Verification items for the finished model (mm, model axes). A direction names the side the tool comes from. Give positions to 0.01 mm unless a question says otherwise; leave off trailing zeros. Write each loop counter-clockwise with the first axis right and the second up, starting at its lowest first coordinate (ties: lowest second). Pieces come first, ordered by that corner, then holes.
from build123d import *

# Parameters (mm, degrees)
SKETCH1_W           = 38
SKETCH1_H           = 22
BOSS_EXTRUDE1_DEPTH = 18
FILLET1_R           = 5
BOSS_EXTRUDE2_DEPTH = 15
BOSS_EXTRUDE3_DEPTH = 13
FILLET2_R           = 2
SKETCH5_R           = 3
SKETCH5_R_2         = 1.5
CUT_EXTRUDE1_DEPTH  = 52.516987581


with BuildPart() as part:
    # Sketch1 → Boss-Extrude1 (new body)
    with BuildSketch(Plane(origin=(0, 0, 0), x_dir=(0, 0, -1), z_dir=(1, 0, 0))):
        Rectangle(SKETCH1_W, SKETCH1_H)
    extrude(amount=BOSS_EXTRUDE1_DEPTH)

    # Fillet1
    fillet1_edges = [part.edges().sort_by_distance(p)[0] for p in [
        (9, 11, 19),
        (9, -11, 19),
    ]]
    fillet(fillet1_edges, radius=FILLET1_R)

    # Sketch3 → Boss-Extrude2 (add)
    with BuildSketch(Plane(origin=(0, 0, -19), x_dir=(-1, 0, 0), z_dir=(0, 0, -1))):
        with BuildLine():
            Line((-18, 6.32455532), (-18, -6.32455532))
            ThreePointArc((-18, -6.32455532), (-9, -11), (0, -6.32455532))
            Line((0, -6.32455532), (0, 6.32455532))
            ThreePointArc((0, 6.32455532), (-9, 11), (-18, 6.32455532))
        make_face()
    extrude(amount=BOSS_EXTRUDE2_DEPTH)

    # Sketch4 → Boss-Extrude3 (add)
    with BuildSketch(Plane(origin=(0, 0, -34), x_dir=(-1, 0, 0), z_dir=(0, 0, -1))):
        with BuildLine():
            Line((-17, 6), (-17, -6))
            ThreePointArc((-17, -6), (-9, -10), (-1, -6))
            Line((-1, -6), (-1, 6))
            ThreePointArc((-1, 6), (-9, 10), (-17, 6))
        make_face()
    extrude(amount=BOSS_EXTRUDE3_DEPTH)

    # Fillet2
    fillet2_edges = [part.edges().sort_by_distance(p)[0] for p in [
        (9, 10, -47),
        (9, -10, -47),
    ]]
    fillet(fillet2_edges, radius=FILLET2_R - 0.0001)  # a hair under: the kernel refuses the full size

    # Sketch5 → Cut-Extrude1 (cut, through all)
    with BuildSketch(Plane(origin=(18, 0, 0), x_dir=(0, 0, -1), z_dir=(1, 0, 0))):
        with Locations((-8, 0)):
            Circle(SKETCH5_R)
        with Locations((14, -9)):
            Circle(SKETCH5_R_2)
        with Locations(Location((14, 9, 0), (0, 0, 180))):
            Circle(SKETCH5_R_2)
    extrude(amount=-CUT_EXTRUDE1_DEPTH, mode=Mode.SUBTRACT)


solid = part.part
Item 1: Release check for a two-part mould opening along Y. For faces 5 (the face through (9, 11, -26)), 6 (the face through (9.1, -9.9, -12.8)), 7 (the face through (2, -10, -19)) record: released by +Y, released by -Y, zero draft, split by the parting line, or undercut.
Answer key:
face 5: released by +Y
face 6: undercut
face 7: zero draft
Item 2: Sectioned sample at D-D on z = -24. Record the cut outline in (x, y), then the cut area to 3 significant figures.
Answer key:
outline: (0, -6.32) arc R11 ccw to (18, -6.32) - (18, 6.32) arc R11 ccw to (0, 6.32) - close
area: 346 mm2
Item 3: Sectioned sample at A-A on z = 8. Record the cut outline in (x, y).
Answer key:
outline: (0, -11) - (18, -11) - (18, -3) - (0, -3) - close; (0, 3) - (18, 3) - (18, 11) - (0, 11) - close
Item 4: Depth check by flat-ended pin: pin 1 (2.5 mm diameter, centred on x = 13, y = -8.5, fed in from -Z); pin 2 (1.4 mm diameter, centred on x = 6, y = 9, fed in from -Z); pin 3 (5 mm diameter, centred on x = 14, y = -7.5, fed in from +Z); pin 4 (4 mm diameter, centred on x = 4, z = -30.5, fed in from +Y). Enter the tip coordinate at first touch or a pass-through.
Answer key:
pin 1: stops at z = -46.99
pin 2: stops at z = -46.84
pin 3: stops at z = 19
pin 4: stops at y = 10.58
Item 5: Sectioned sample at B-B on z = -14. Record the cut outline in (x, y).
Answer key:
outline: (0, -11) - (18, -11) - (18, -10.5) - (0, -10.5) - close; (0, -7.5) - (18, -7.5) - (18, 7.5) - (0, 7.5) - close; (0, 10.5) - (18, 10.5) - (18, 11) - (0, 11) - close
Item 6: Set-up check for faces 1 (the face through (17, 0, -40)), 2 (the face through (1, 0, -40)), 3 (the face through (16, 10, -19)), 4 (the face through (9, -11, -26)): record each of +Z, -Z, +X, -X, +Y, -Y from which the full face is reachable in a straight line by a thin tool's end or side.
Answer key:
face 1: -Z, +X, +Y, -Y
face 2: -Z, -X, +Y, -Y
face 3: -Z, +X, +Y
face 4: -Z, -Y
Item 7: Scan lines: line 1 along Y through (x, z) = (7.25, -14); line 2 along Y through (x, z) = (11.5, 8); line 3 along Z through (x, y) = (4.5, 9). Record each from-to range of solid material in increasing order.
Answer key:
line 1: y = -11 to -10.5, -7.5 to 7.5, 10.5 to 11
line 2: y = -11 to -3, 3 to 11
line 3: z = -34 to -15.5, -12.5 to 18
Item 8: Sectioned sample at C-C on x = 7.5. State how many separate pieces and enclosed holes the cut face has, then the cut area to 3 significant figures.
Answer key:
separate pieces: 1
enclosed holes: 3
area: 1,370 mm2
